```python
from build123d import *

# Parameters (mm, degrees)
BOSS_EXTRU_1_DEPTH      = 5
ESQUISSE9_W             = 5
ESQUISSE9_H             = 5
BOSS_EXTRU_3_DEPTH      = 40
ESQUISSE11_R            = 1.009332427
ENL_V_MAT_EXTRU_2_DEPTH = 40
CONG_1_R                = 3
CONG_2_R                = 3


with BuildPart() as part:
    # Esquisse1 → Boss.-Extru.1 (new body)
    with BuildSketch(Plane.XY):
        with BuildLine():
            Line((26.025021052, -0.447992933), (-24.829805977, 87.508811894))
            Line((-24.829805977, 87.508811894), (-24.829805977, 1.293439737))
            ThreePointArc((-24.829805977, 1.293439737), (1.080284786, 14.518282983), (26.025021052, -0.447992933))
        make_face()
    extrude(amount=BOSS_EXTRU_1_DEPTH)

    # Esquisse9 → Boss.-Extru.3 (add)
    with BuildSketch(Plane(origin=(0, 87.489884498, 0), x_dir=(1, 0, 0), z_dir=(0, 1, 0))):
        with Locations((-27.329805977, -2.5)):
            Rectangle(ESQUISSE9_W, ESQUISSE9_H)
    extrude(amount=-BOSS_EXTRU_3_DEPTH)

    # Esquisse11 → Enlèv. mat.-Extru.2 (cut)
    with BuildSketch(Plane(origin=(0, 87.489884498, 0), x_dir=(1, 0, 0), z_dir=(0, 1, 0))):
        with Locations(Location((-27.353173819, -2.5, 0), (0, 0, 270))):
            Circle(ESQUISSE11_R)
    extrude(amount=-ENL_V_MAT_EXTRU_2_DEPTH, mode=Mode.SUBTRACT)

    # Congé1
    cong_1_edges = [part.edges().sort_by_distance(p)[0] for p in [
        (-29.829805977, 67.489884498, 0),
    ]]
    fillet(cong_1_edges, radius=CONG_1_R)

    # Congé2
    # the kernel refuses this fillet: 3 mm, written as the material it takes off along each edge
    with BuildSketch(Plane(origin=(-29.829805977, 94.56095231, 5), x_dir=(0, 0, -1), z_dir=(0, -1, 0))) as cong_2_piece_1:
        with BuildLine():
            CenterArc((3, 2.828427125), CONG_2_R, 180, 70.528779366)
            Line((0, 2.828427125), (-0.06, 2.828427125))
            Line((-0.06, 2.828427125), (-0.06, 0))
            Line((-0.06, 0), (0, -0.06))
            ThreePointArc((0, -0.06), (1, -0.06), (1.98, -0.056568542))
            Line((1.98, -0.056568542), (2, 0))
        make_face()
    extrude(amount=54.142135624, mode=Mode.SUBTRACT)


solid = part.part
```
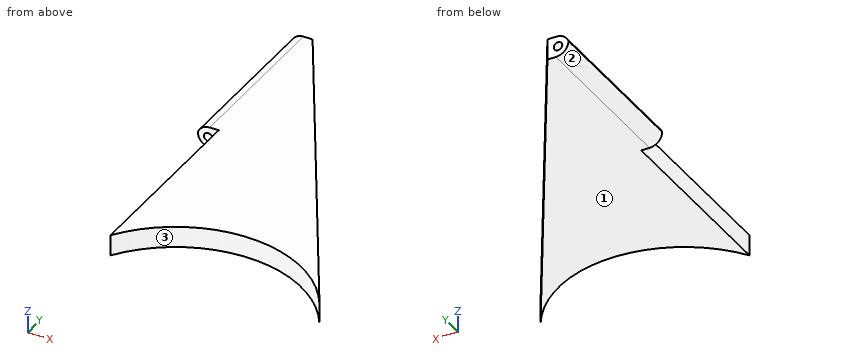
Geometry check sheet. Reference: the model listing, model coordinates, mm. Face numbers are marked on the shaded views. Give positions to 0.01 mm unless a question says otherwise; leave off trailing zeros. Loops run counter-clockwise (first coordinate to the right, second up) from the corner with the lowest first, then second, coordinate; pieces in that order, holes last. Notation, with made-up numbers: M 34.5,-21.75 L 87.5,-21.75 A25 cw 87.5,11.25 Z; hole C -26,64.25 d7. An arc over 180 degrees is marked long. Write item = value, one per line.
(1) Gauge pin test, flat ends, axial feed: pin 1 Ø2 at (y, z) = (23, 2) entering from -X; pin 2 Ø2.5 at (x, z) = (-27.35, 2.5) entering from -Y; pin 3 Ø1.5 at (x, z) = (17.5, 3.5) entering from +Y. Record the tip position at first contact, or that the pin passes through.
Answer below:
pin_1 = -24.83
pin_2 = 47.49
pin_3 = 15.59
(2) Material ranges on line 1 (X direction, y = 64, z = 2.5); line 2 (X direction, y = 73, z = 2.75); line 3 (X direction, y = 38.5, z = 2.9), recorded low to high. Write a range as [from, to].
Answer below:
line_1 = [-29.79, -28.36], [-26.34, -11.24]
line_2 = [-29.82, -28.33], [-26.38, -16.44]
line_3 = [-24.83, 3.51]
(3) Release check for a two-part mould opening along X. For the marked faces 1, 2 and 3 record: released by +X, released by -X, zero draft, split by the parting line, or undercut.
Answer below:
face_1 = zero draft
face_2 = released by -X
face_3 = undercut
(4) Sectioned sample at B-B, the plane y = 61. Record the cut outline in (x, z).
Answer below:
outline = M -29.83,3 A3 ccw -26.83,0 L -9.5,0 L -9.5,5 L -27,5 A3 ccw Z; hole C -27.35,2.5 d2.02
(5) Sectioned sample at A-A, the plane y = 13. Record the cut outline in (x, z).
Answer below:
outline = M -24.83,0 L -9.42,0 L -9.42,5 L -24.83,5 Z; M 9.53,0 L 18.25,0 L 18.25,5 L 9.53,5 Z
(6) Sectioned sample at C-C, the plane x = -5. Record the cut outline in (y, z).
Answer below:
outline = M 14.11,0 L 53.21,0 L 53.21,5 L 14.11,5 Z
(7) Sectioned sample at D-D, the plane y = 45.5. Record the cut outline in (x, z), plus the area to 3 significant figures.
Answer below:
outline = M -24.83,0 L -0.54,0 L -0.54,5 L -24.83,5 Z
area = 121 mm2
